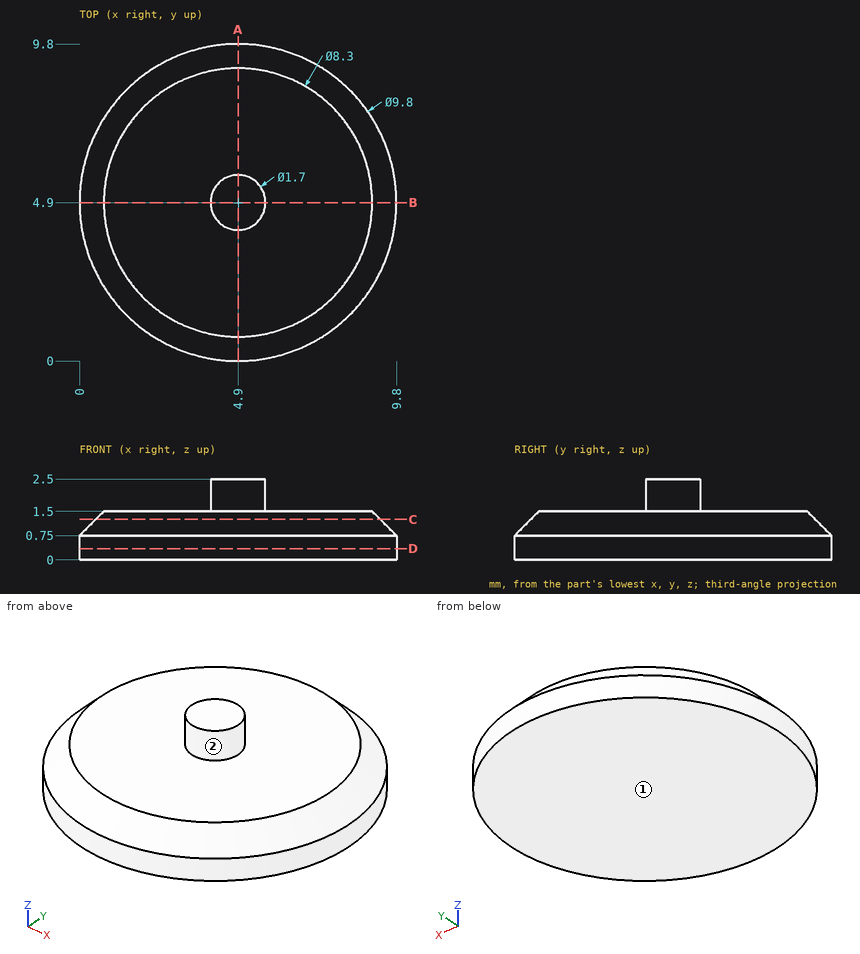
Print and shaded views of the part. All mm, measured from the part's lowest x, y and z. A direction names the side the tool comes from. Give positions to 0.01 mm unless a question says otherwise; leave off trailing zeros. Write each loop counter-clockwise with the first axis right and the second up, starting at its lowest first coordinate (ties: lowest second). Pieces come first, ordered by that corner, then holes. Notation, with made-up numbers: M 52,-9 L 100,-9 A13 cw 100,1 Z; hole C 42.5,85.5 d4. An arc over 180 degrees is marked long. Use a Markdown table: item, result.
1) Drill centre lines: line 1 (X direction, y = 7.5, z = 0.35); line 2 (Z direction, x = 5.25, y = 3); line 3 (X direction, y = 7, z = 0.9). Where is each one in solid material? Low to high. Write a range as from..to.
Responses:
| item | result |
|---|---|
| line 1 | x = 0.75..9.05 |
| line 2 | z = 0..1.5 |
| line 3 | x = 0.64..9.16 |
2) Cut at C-C (z = 1.25). List the corners of the cut face in (x, y).
Responses:
| item | result |
|---|---|
| outline | C 4.9,4.9 d8.8 |
3) Cut at A-A (x = 4.9). List the corners of the cut face in (y, z).
Responses:
| item | result |
|---|---|
| outline | M 0,0 L 9.8,0 L 9.8,0.75 L 9.05,1.5 L 5.75,1.5 L 5.75,2.5 L 4.05,2.5 L 4.05,1.5 L 0.75,1.5 L 0,0.75 Z |
4) Pin check, flat tips, straight feed: pin 1 (5 mm diameter, centred on x = 8, y = 6.5, fed in from -Z); pin 2 (1.5 mm diameter, centred on x = 6.5, z = 2, fed in from +Y); pin 3 (1 mm diameter, centred on x = 8.5, z = 1.5, fed in from -Y). Stop position of each tip, or through.
Responses:
| item | result |
|---|---|
| pin 1 | stops at z = 0 |
| pin 2 | stops at y = 9.04 |
| pin 3 | stops at y = 1.77 |
5) Tool access for the marked faces 1 and 2: list every direction of +Z, -Z, +X, -X, +Y, -Y with a clear straight run to the whole face (end or side of a thin tool).
Responses:
| item | result |
|---|---|
| face 1 | -Z, +X, -X, +Y, -Y |
| face 2 | +Z |
6) Cut at D-D (z = 0.35). List the corners of the cut face in (x, y).
Responses:
| item | result |
|---|---|
| outline | C 4.9,4.9 d9.8 |
